```python
from build123d import *

# Parameters (mm, degrees)
SKETCH1_W           = 120
SKETCH1_H           = 140
SKETCH1_R           = 2.6
SKETCH1_R_2         = 3.55
BOSS_EXTRUDE1_DEPTH = 3.2
FILLET1_R           = 10


with BuildPart() as part:
    # Sketch1 → Boss-Extrude1 (new body)
    with BuildSketch(Plane.XY):
        Rectangle(SKETCH1_W, SKETCH1_H)
        Circle(SKETCH1_R, mode=Mode.SUBTRACT)
        with Locations((10, 0)):
            Circle(SKETCH1_R, mode=Mode.SUBTRACT)
        with Locations((20, 0)):
            Circle(SKETCH1_R, mode=Mode.SUBTRACT)
        with Locations((30, 0)):
            Circle(SKETCH1_R, mode=Mode.SUBTRACT)
        with Locations((-10, 0)):
            Circle(SKETCH1_R, mode=Mode.SUBTRACT)
        with Locations((-20, 0)):
            Circle(SKETCH1_R, mode=Mode.SUBTRACT)
        with Locations((-30, 0)):
            Circle(SKETCH1_R, mode=Mode.SUBTRACT)
        with Locations((0, 10)):
            Circle(SKETCH1_R, mode=Mode.SUBTRACT)
        with Locations((0, 20)):
            Circle(SKETCH1_R, mode=Mode.SUBTRACT)
        with Locations((0, 30)):
            Circle(SKETCH1_R, mode=Mode.SUBTRACT)
        with Locations((0, -10)):
            Circle(SKETCH1_R, mode=Mode.SUBTRACT)
        with Locations((0, -20)):
            Circle(SKETCH1_R, mode=Mode.SUBTRACT)
        with Locations((0, -30)):
            Circle(SKETCH1_R, mode=Mode.SUBTRACT)
        with Locations((42.3, 0)):
            Circle(SKETCH1_R, mode=Mode.SUBTRACT)
        with Locations((-42.3, 0)):
            Circle(SKETCH1_R_2, mode=Mode.SUBTRACT)
        with Locations((-42.3, 26.15)):
            Circle(SKETCH1_R_2, mode=Mode.SUBTRACT)
        with Locations((-42.3, 52.3)):
            Circle(SKETCH1_R_2, mode=Mode.SUBTRACT)
        with Locations((-42.3, -26.15)):
            Circle(SKETCH1_R_2, mode=Mode.SUBTRACT)
        with Locations((-42.3, -52.3)):
            Circle(SKETCH1_R_2, mode=Mode.SUBTRACT)
        with Locations((42.3, 26.15)):
            Circle(SKETCH1_R, mode=Mode.SUBTRACT)
        with Locations((42.3, 52.3)):
            Circle(SKETCH1_R, mode=Mode.SUBTRACT)
        with Locations((42.3, -26.15)):
            Circle(SKETCH1_R, mode=Mode.SUBTRACT)
        with Locations((42.3, -52.3)):
            Circle(SKETCH1_R, mode=Mode.SUBTRACT)
        with Locations((-32.3, 52.3)):
            Circle(SKETCH1_R_2, mode=Mode.SUBTRACT)
        with Locations((-22.3, 52.3)):
            Circle(SKETCH1_R_2, mode=Mode.SUBTRACT)
        with Locations((-32.3, -52.3)):
            Circle(SKETCH1_R_2, mode=Mode.SUBTRACT)
        with Locations((-22.3, -52.3)):
            Circle(SKETCH1_R_2, mode=Mode.SUBTRACT)
        with Locations((32.3, 52.3)):
            Circle(SKETCH1_R, mode=Mode.SUBTRACT)
        with Locations((22.3, 52.3)):
            Circle(SKETCH1_R, mode=Mode.SUBTRACT)
        with Locations((32.3, -52.3)):
            Circle(SKETCH1_R, mode=Mode.SUBTRACT)
        with Locations((22.3, -52.3)):
            Circle(SKETCH1_R, mode=Mode.SUBTRACT)
        with Locations((0, 52.3)):
            Circle(SKETCH1_R, mode=Mode.SUBTRACT)
        with Locations((10, 52.3)):
            Circle(SKETCH1_R, mode=Mode.SUBTRACT)
        with Locations((-10, 52.3)):
            Circle(SKETCH1_R, mode=Mode.SUBTRACT)
        with Locations((-20, 30)):
            Circle(SKETCH1_R, mode=Mode.SUBTRACT)
        with Locations((20, 30)):
            Circle(SKETCH1_R, mode=Mode.SUBTRACT)
        with Locations((-30, 20)):
            Circle(SKETCH1_R, mode=Mode.SUBTRACT)
        with Locations((30, 20)):
            Circle(SKETCH1_R, mode=Mode.SUBTRACT)
        with Locations((-45, 10)):
            Circle(SKETCH1_R, mode=Mode.SUBTRACT)
        with Locations((45, 10)):
            Circle(SKETCH1_R, mode=Mode.SUBTRACT)
        with Locations((45, -10)):
            Circle(SKETCH1_R, mode=Mode.SUBTRACT)
        with Locations((30, -20)):
            Circle(SKETCH1_R, mode=Mode.SUBTRACT)
        with Locations((20, -30)):
            Circle(SKETCH1_R, mode=Mode.SUBTRACT)
        with Locations((10, -52.3)):
            Circle(SKETCH1_R, mode=Mode.SUBTRACT)
        with Locations((0, -52.3)):
            Circle(SKETCH1_R, mode=Mode.SUBTRACT)
        with Locations((-10, -52.3)):
            Circle(SKETCH1_R, mode=Mode.SUBTRACT)
        with Locations((-20, -30)):
            Circle(SKETCH1_R, mode=Mode.SUBTRACT)
        with Locations((-30, -20)):
            Circle(SKETCH1_R, mode=Mode.SUBTRACT)
        with Locations((-45, -10)):
            Circle(SKETCH1_R, mode=Mode.SUBTRACT)
    extrude(amount=-BOSS_EXTRUDE1_DEPTH)

    # Fillet1
    fillet1_edges = [part.edges().sort_by_distance(p)[0] for p in [
        (60, -70, -1.6),
        (-60, -70, -1.6),
        (-60, 70, -1.6),
        (60, 70, -1.6),
    ]]
    fillet(fillet1_edges, radius=FILLET1_R)


solid = part.part
```
Design review of the part built by this model. Coordinates are the model's own, in mm. Coordinates: 2 decimals unless noted, no trailing zeros. Order: outer loops, then holes, each group sorted by start corner. A loop starts at its lowest first (then second) coordinate and runs counter-clockwise, first axis right, second up. Notation, with made-up numbers: (80.25, -6.5) - (101.25, -6.5) arc R14 ccw to (101.25, 5.5) - close; hole circle Ø10 at (2.5, 38). An arc over 180 degrees is marked (long way). Answer in a Markdown table with one row per item.
(1) Clearance check with a flat-ended pin moving along its axis: pin 1 (8.5 mm diameter, centred on x = 10, y = -52.3, fed in from -Z). State where the tip first meets the part, or that it passes through.
Checked values:
| item | result |
|---|---|
| pin 1 | z = -3.2 |
(2) Consider section B-B on y = 0. Give the number of separate pieces and of enclosed holes in the cut face, plus the area to 3 significant figures.
Checked values:
| item | result |
|---|---|
| separate pieces | 10 |
| enclosed holes | 0 |
| area | 228 mm^2 |
(3) Wall thickness on line 1 along Y through (x, z) = (20, -1.4); line 2 along Y through (x, z) = (-22, -2.5); line 3 along X through (y, z) = (-28, -0.3): over which ranges is each line inside the solid? List them lowest first. Write a range as from..to.
Checked values:
| item | result |
|---|---|
| line 1 | -70..-53.51, -51.09..-32.6, -27.4..-2.6, 2.6..27.4, 32.6..51.09, 53.51..70 |
| line 2 | -70..-55.84, -48.76..-31.66, -28.34..-1.66, 1.66..28.34, 31.66..48.76, 55.84..70 |
| line 3 | -60..-45.33, -39.27..-21.66, -18.34..-1.66, 1.66..18.34, 21.66..40.47, 44.13..60 |
(4) Consider section A-A on y = -20. State the section outline as (x, z) points, plus the area to 3 significant figures.
Checked values:
| item | result |
|---|---|
| outline | (-60, -3.2) - (-32.6, -3.2) - (-32.6, 0) - (-60, 0) - close; (-27.4, -3.2) - (-2.6, -3.2) - (-2.6, 0) - (-27.4, 0) - close; (2.6, -3.2) - (27.4, -3.2) - (27.4, 0) - (2.6, 0) - close; (32.6, -3.2) - (60, -3.2) - (60, 0) - (32.6, 0) - close |
| area | 334 mm^2 |
